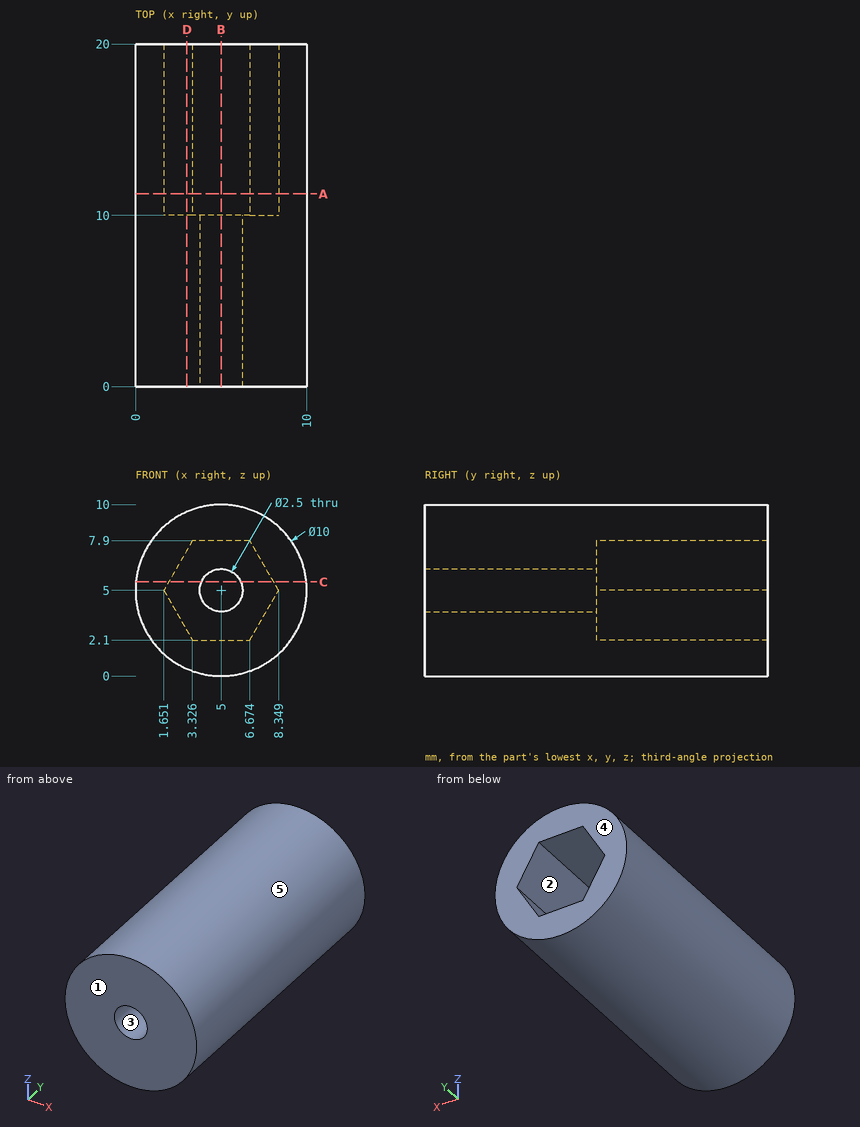
Geometry check sheet. Reference: drawing and pictorial views, mm from the part's lowest x, y, z. A direction names the side the tool comes from. Round coordinates to 2 decimals unless told otherwise and drop trailing zeros. Order: outer loops, then holes, each group sorted by start corner. A loop starts at its lowest first (then second) coordinate and runs counter-clockwise, first axis right, second up. Notation, with made-up numbers: (25, 4) - (49, 4) arc R29 ccw to (49, 41) - close; hole circle Ø10 at (89, 11.25). An arc over 180 degrees is marked (long way). Write item = value, one per line.
Q1. Go/stop test with flat-tipped pins: pin 1 (1.7 mm diameter, centred on x = 4.5, y = 17.5, fed in from -Z); pin 2 (2 mm diameter, centred on x = 4, z = 5, fed in from +Y). Record where each tip stops, or that it passes through.
Computed:
pin_1 = 0
pin_2 = 10
Q2. Section check A-A (y = 11.25). Record the boundary of the cut face in (x, z) (1 decimal), and give its area (3 significant figures).
Computed:
outline = circle Ø10 at (5, 5); hole (1.7, 5) - (3.3, 2.1) - (6.7, 2.1) - (8.3, 5) - (6.7, 7.9) - (3.3, 7.9) - close
area = 49.4 mm^2
Q3. Thickness scan on line 1 along Z through (x, y) = (5, 3.5); line 2 along X through (y, z) = (12.75, 4); line 3 along X through (y, z) = (19, 5.75) (1 decimal). Record the ranges inside material, lowest first.
Computed:
line_1 = 0 to 3.75, 6.25 to 10
line_2 = 0.1 to 2.23, 7.77 to 9.9
line_3 = 0.1 to 2.1, 7.9 to 9.9
Q4. Section check C-C (z = 5.5). Record the boundary of the cut face in (x, y) (1 decimal).
Computed:
outline = (0, 0) - (3.9, 0) - (3.9, 10) - (1.9, 10) - (1.9, 20) - (0, 20) - close; (6.1, 0) - (10, 0) - (10, 20) - (8.1, 20) - (8.1, 10) - (6.1, 10) - close
Q5. Section check D-D (x = 3). Record the boundary of the cut face in (y, z), and give its area (3 significant figures).
Computed:
outline = (0, 0.42) - (20, 0.42) - (20, 2.66) - (10, 2.66) - (10, 7.34) - (20, 7.34) - (20, 9.58) - (0, 9.58) - close
area = 137 mm^2
Q6. Draft check along X on the marked faces 3, 4 and 5. Enter one of: pulls with the +X half, pulls with the -X half, needs draft (parallel to the pull), parting line crosses it, or undercut.
Computed:
face_3 = undercut
face_4 = needs draft
face_5 = parting line crosses it
Q7. Section check B-B (x = 5). Record the boundary of the cut face in (y, z), and give its area (3 significant figures).
Computed:
outline = (0, 0) - (20, 0) - (20, 2.1) - (10, 2.1) - (10, 3.75) - (0, 3.75) - close; (0, 6.25) - (10, 6.25) - (10, 7.9) - (20, 7.9) - (20, 10) - (0, 10) - close
area = 117 mm^2
Q8. Tool access check on the marked faces 1 and 2. Record the directions out of +Z, -Z, +X, -X, +Y, -Y that give a thin tool (end or side, any length) a straight path to the whole face; none if there is none.
Computed:
face_1 = +Z, -Z, +X, -X, -Y
face_2 = +Y
